Could you check a few things on this drawing? It's one solid part, dimensions in mm from its lowest x, y, z. Round coordinates to 2 decimals unless told otherwise and drop trailing zeros. Write each loop counter-clockwise with the first axis right and the second up, starting at its lowest first coordinate (ties: lowest second). Pieces come first, ordered by that corner, then holes. Notation, with made-up numbers: (7, 88) -> (64, 88) arc R27 ccw to (64, 127) -> close; hole circle Ø11 at (15.5, 61.25). An arc over 180 degrees is marked (long way). Return JSON: item names as keys, results as strings.
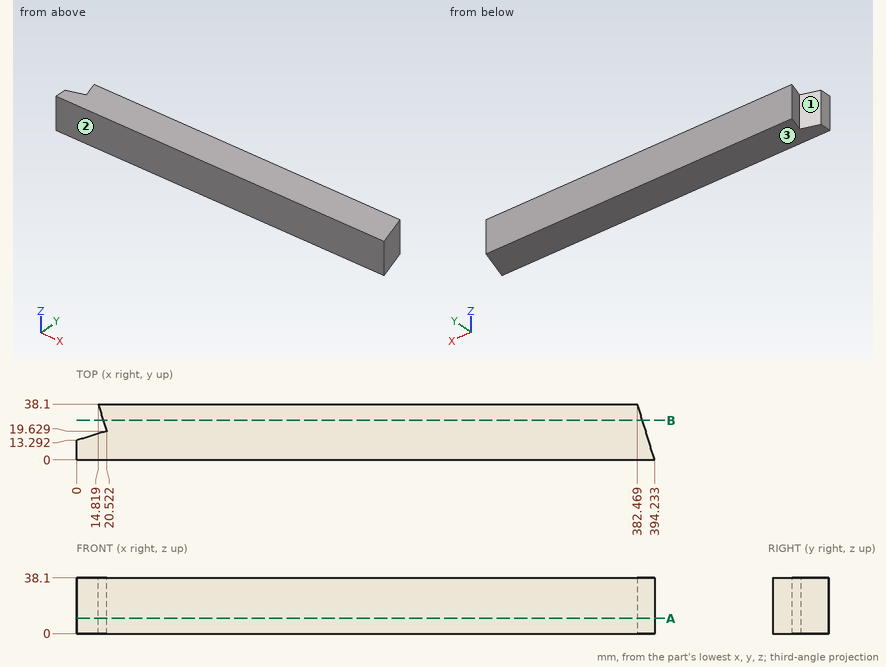
1) If I drill on probe 1 along X at (y, z) = (21, 18.5); probe 2 along X at (y, z) = (35.5, 24), over which ranges is the centre line in solid material (lowest first)? Write a range as [from, to].
Return value:
{"probe 1": "[20.1, 387.75]", "probe 2": "[15.62, 383.27]"}
2) I want a section at A-A, the plane z = 10.5. Please give me the cut outline in (x, y).
Return value:
{"outline": "(0, 0) -> (394.23, 0) -> (382.47, 38.1) -> (14.82, 38.1) -> (20.52, 19.63) -> (0, 13.29) -> close"}
3) Thinking about a two-plate mould opening in Y: for the marked faces 1, 2 and 3, which applies, pulls with the +Y half, pulls with the -Y half, needs draft (parallel to the pull), parting line crosses it, or undercut?
Return value:
{"face 1": "undercut", "face 2": "pulls with the -Y half", "face 3": "needs draft"}
4) Will these pins go through, and if not, where does the flat tip stop? pin 1 Ø10 at (y, z) = (18, 5) entering from +X; pin 2 Ø1.5 at (x, z) = (260.5, 28.5) entering from -Y; pin 3 Ø10 at (y, z) = (6, 27) entering from +X (1 decimal).
Return value:
{"pin 1": "x = 390.22", "pin 2": "y = 0", "pin 3": "x = 393.9"}
5) I want a section at B-B, the plane y = 27. Please give me the cut outline in (x, z).
Return value:
{"outline": "(18.25, 0) -> (385.9, 0) -> (385.9, 38.1) -> (18.25, 38.1) -> close"}
